```python
from build123d import *

# Parameters (mm, degrees)
F1_DEPTH = 10


with BuildPart() as f1:
    # F0 (on Top) → F1 (new body)
    with BuildSketch(Plane.XY):
        with BuildLine():
            Line((30, -21.8), (0, -21.8))
            add(Edge.make_bspline(
                [(0, -21.8), (-1.6334013165, -19.5362873508), (-5.3511473255, -17.9243908717), (-12.5395497227, -19.7618053971), (-18.5, -21.8)],
                knots=[0, 0, 0, 0, 0.3971734047, 1, 1, 1, 1], degree=3))
            Line((-18.5, -21.8), (-18.5, -24.8))
            Line((-18.5, -24.8), (0, -24.8))
            Line((0, -24.8), (30.0251226872, -24.8))
            ThreePointArc((30.0251226872, -24.8), (54.8251226872, 0), (30.0251226872, 24.8))
            Line((30.0251226872, 24.8), (0, 24.8))
            Line((0, 24.8), (-18.5, 24.8))
            Line((-18.5, 24.8), (-18.5, 21.8))
            add(Edge.make_bspline(
                [(0, 21.8), (-1.6334013165, 19.5362873508), (-5.3511473255, 17.9243908717), (-12.5395497227, 19.7618053971), (-18.5, 21.8)],
                knots=[0, 0, 0, 0, 0.3971734047, 1, 1, 1, 1], degree=3))
            Line((0, 21.8), (30, 21.8))
            ThreePointArc((30, 21.8), (51.8, 0), (30, -21.8))
        make_face()
    extrude(amount=F1_DEPTH)


solid = f1.part
```
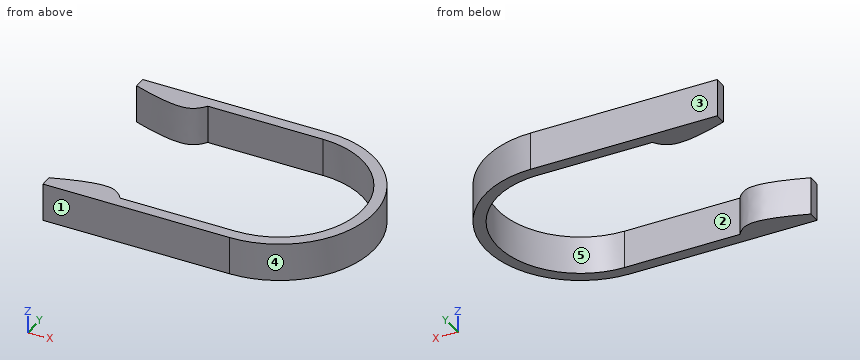
Read the model definition and answer for the solid it produces. Units are mm, in the model's axes. Face numbers are marked on the shaded views. A direction names the side the tool comes from. Give positions to 0.01 mm unless a question says otherwise; leave off trailing zeros. Loops run counter-clockwise (first coordinate to the right, second up) from the corner with the lowest first, then second, coordinate; pieces in that order, holes last.
Item 1: For the marked faces 4 and 5, determine the directions among +Z, -Z, +X, -X, +Y, -Y from which every point of the face is accessible in a straight line to the end or side of a thin tool.
Item 2: Each of these flat-tipped pins is pushed along its axis until it touches: pin 1 Ø3 at (x, z) = (46.5, 6.5) entering from -Y; pin 2 Ø5 at (y, z) = (-8.5, 5.5) entering from +X; pin 3 Ø3 at (y, z) = (6, 5.5) entering from +X. Where does it stop, or does it pass through?
Item 3: Find the intervals of material crossed by line 1 along Y through (x, z) = (18.5, 7.5); line 2 along Y through (x, z) = (-5.5, 1.25); line 3 along X through (y, z) = (0, 8.5), in increasing order.
Item 4: The part is cut by section A-A (x = 23.5). Write down the section's boundary in (y, z).
Item 5: The part is cut by section B-B (y = 0). Write down the section's boundary in (x, z), and give its area (3 significant figures).
Item 6: The mould has two halves that part along Y. Classify the marked faces 1, 2 and 3: released by +Y, released by -Y, zero draft, split by the parting line, or undercut.
Item 7: The part is cut by section C-C (y = -16). Write down the section's boundary in (x, z), and give its area (3 significant figures).
Taken from the geometry:
1. face 4: +Z, -Z, +X
1. face 5: +Z, -Z
2. pin 1: stops at y = -19.77
2. pin 2: stops at x = 54.09
2. pin 3: stops at x = 54.41
3. line 1: y = -24.8 to -21.8, 21.8 to 24.8
3. line 2: y = -24.8 to -18.79, 18.79 to 24.8
3. line 3: x = 51.8 to 54.83
4. outline: (-24.8, 0) - (-21.8, 0) - (-21.8, 10) - (-24.8, 10) - close; (21.8, 0) - (24.8, 0) - (24.8, 10) - (21.8, 10) - close
5. outline: (51.8, 0) - (54.83, 0) - (54.83, 10) - (51.8, 10) - close
5. area: 30.3 mm2
6. face 1: released by -Y
6. face 2: undercut
6. face 3: released by +Y
7. outline: (44.81, 0) - (48.97, 0) - (48.97, 10) - (44.81, 10) - close
7. area: 41.7 mm2
